The model under review builds one solid part; all positions refer to its coordinate system, in mm. Face numbers are marked on the shaded views. A direction names the side the tool comes from. Round coordinates to 2 decimals unless told otherwise and drop trailing zeros. Write each loop counter-clockwise with the first axis right and the second up, starting at its lowest first coordinate (ties: lowest second). Pieces come first, ordered by that corner, then holes. Notation, with made-up numbers: (-14.75, -16.5) - (43.25, -16.5) arc R22 cw to (43.25, 22.5) - close; hole circle Ø3 at (84, 11.5). An arc over 180 degrees is marked (long way). Return JSON: item names as keys, results as strings.
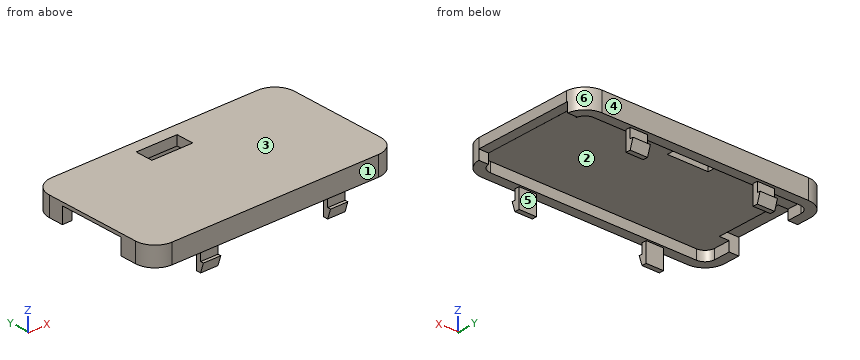
from build123d import *

# Parameters (mm, degrees)
EXTRUDE_1_DEPTH     = 1.5
EXTRUDE_2_DEPTH     = 1.5
CUT_EXTRUDE_2_DEPTH = 1.5
SKETCH_8_W          = 6.342405544
SKETCH_8_H          = 2.722912939
CUT_EXTRUDE_3_DEPTH = 1.5
SKETCH_9_W          = 2.696269273
SKETCH_9_H          = 0.7312398
EXTRUDE_4_DEPTH     = 3
EXTRUDE_6_REACH     = 61.436
CUT_EXTRUDE_4_DEPTH = 17.033846789
SKETCH_6_W          = 3.802870335
SKETCH_6_H          = 10.25
CUT_EXTRUDE_5_DEPTH = 3.024817901


with BuildPart() as part:
    # 草图1 → 凸台-拉伸1 (new body)
    with BuildSketch(Plane.XY.offset(46.24708128)):
        with BuildLine():
            Line((-18.935673231, -7.132078693), (13.064326769, -7.132078693))
            ThreePointArc((13.064326769, -7.132078693), (15.140982735, -6.297142202), (16.061721471, -4.257078693))
            Line((16.061721471, -4.257078693), (16.061721471, 10.992921307))
            ThreePointArc((16.061721471, 10.992921307), (15.140982735, 13.032984817), (13.064326769, 13.867921307))
            Line((13.064326769, 13.867921307), (-18.935673231, 13.867921307))
            ThreePointArc((-18.935673231, 13.867921307), (-21.056993574, 12.989241651), (-21.935673231, 10.867921307))
            Line((-21.935673231, 10.867921307), (-21.935673231, -4.132078693))
            ThreePointArc((-21.935673231, -4.132078693), (-21.056993574, -6.253399036), (-18.935673231, -7.132078693))
        make_face()
        with BuildLine():
            Line((13.064326769, -5.632078693), (-18.935673231, -5.632078693))
            ThreePointArc((-18.935673231, -5.632078693), (-19.996333403, -5.192738865), (-20.435673231, -4.132078693))
            Line((-20.435673231, -4.132078693), (-20.435673231, 10.867921307))
            ThreePointArc((-20.435673231, 10.867921307), (-19.996333403, 11.928581479), (-18.935673231, 12.367921307))
            Line((-18.935673231, 12.367921307), (13.064326769, 12.367921307))
            ThreePointArc((13.064326769, 12.367921307), (14.124986941, 11.928581479), (14.564326769, 10.867921307))
            Line((14.564326769, 10.867921307), (14.564326769, -4.132078693))
            ThreePointArc((14.564326769, -4.132078693), (14.124986941, -5.192738865), (13.064326769, -5.632078693))
        make_face(mode=Mode.SUBTRACT)
    extrude(amount=EXTRUDE_1_DEPTH)

    # 草图4 → 凸台-拉伸2 (add)
    with BuildSketch(Plane.XY.offset(47.74708128)):
        with BuildLine():
            Line((-21.935673231, 10.867921307), (-21.935673231, -4.132078693))
            ThreePointArc((-21.935673231, -4.132078693), (-21.056993574, -6.253399036), (-18.935673231, -7.132078693))
            Line((-18.935673231, -7.132078693), (13.064326769, -7.132078693))
            ThreePointArc((13.064326769, -7.132078693), (15.140982735, -6.297142202), (16.061721471, -4.257078693))
            Line((16.061721471, -4.257078693), (16.061721471, 10.992921307))
            ThreePointArc((16.061721471, 10.992921307), (15.140982735, 13.032984817), (13.064326769, 13.867921307))
            Line((13.064326769, 13.867921307), (-18.935673231, 13.867921307))
            ThreePointArc((-18.935673231, 13.867921307), (-21.056993574, 12.989241651), (-21.935673231, 10.867921307))
        make_face()
    extrude(amount=EXTRUDE_2_DEPTH)

    # 草图7 → 切除-拉伸2 (cut)
    with BuildSketch(Plane(origin=(16.061721471, 0, 0), x_dir=(0, 0, -1), z_dir=(1, 0, 0))):
        Polygon((-46.24708128, 11.189366068), (-47.753743169, 11.189366068), (-47.74708128, -4.257078693), (-46.24708128, -4.257078693), align=None)
    extrude(amount=-CUT_EXTRUDE_2_DEPTH, mode=Mode.SUBTRACT)

    # 草图8 → 切除-拉伸3 (cut)
    with BuildSketch(Plane.XY.offset(49.24708128)):
        with Locations((-4.288714371, 10.645412295)):
            Rectangle(SKETCH_8_W, SKETCH_8_H)
    extrude(amount=-CUT_EXTRUDE_3_DEPTH, mode=Mode.SUBTRACT)

    # 草图9 → 凸台-拉伸4 (add)
    with BuildSketch(Plane(origin=(0, 0, 46.24708128), x_dir=(-1, 0, 0), z_dir=(0, 0, -1))):
        with Locations((-6.965713307, 13.038581452)):
            Rectangle(SKETCH_9_W, SKETCH_9_H)
        with Locations((12.764402756, 13.038581452)):
            Rectangle(SKETCH_9_W, SKETCH_9_H)
        with Locations((12.764402756, -6.302738837)):
            Rectangle(SKETCH_9_W, SKETCH_9_H)
        with Locations((-6.965713307, -6.302738837)):
            Rectangle(SKETCH_9_W, SKETCH_9_H)
    extrude(amount=EXTRUDE_4_DEPTH)

    # 凸台-拉伸6: up to this face of the body (flat: up to its plane)
    extrude_6_end = Plane(part.part.faces().sort_by_distance((-14.112537392, 13.038581452, 44.74708128))[0])
    # 草图10 → 凸台-拉伸6 (add, up to the picked face)
    with BuildSketch(Plane(origin=(8.313847943, 0, 0), x_dir=(0, 0, -1), z_dir=(1, 0, 0)), mode=Mode.PRIVATE) as extrude_6_sk1:
        Polygon((-44.74708128, 13.404201352), (-44.74708128, 13.89248872), (-43.24708128, 13.404201352), align=None)
    extrude_6_tool1 = split(extrude(extrude_6_sk1.sketch, amount=-EXTRUDE_6_REACH, mode=Mode.PRIVATE), bisect_by=extrude_6_end, keep=Keep.BOTH, mode=Mode.PRIVATE)
    extrude_6 = extrude_6_tool1.solids().sort_by(Axis((8.313848, 13.566964, 44.247081), (-1, 0, 0)))[0]
    add(extrude_6)

    # 草图11 → 切除-拉伸4 (cut)
    with BuildSketch(Plane(origin=(-11.416268119, 0, 0), x_dir=(0, 0, -1), z_dir=(1, 0, 0))):
        Polygon((-44.74708128, 13.404201352), (-43.24708128, 13.404201352), (-44.74708128, 13.89248872), align=None)
    cut_extrude_4 = extrude(amount=CUT_EXTRUDE_4_DEPTH, mode=Mode.SUBTRACT)

    # 镜向1: 凸台-拉伸6 across plane
    add(extrude_6.mirror(Plane(origin=(0, 3.367921307, 0), x_dir=(0, 0, 1), z_dir=(0, -1, 0))))

    # 镜向2: 切除-拉伸4 across plane
    add(cut_extrude_4.mirror(Plane(origin=(0, 3.367921307, 0), x_dir=(0, 0, 1), z_dir=(0, -1, 0))), mode=Mode.SUBTRACT)

    # 草图6 → 切除-拉伸5 (cut)
    with BuildSketch(Plane.ZY.offset(21.935673231)):
        with Locations((46.829796448, 3.511921307)):
            Rectangle(SKETCH_6_W, SKETCH_6_H)
    extrude(amount=-CUT_EXTRUDE_5_DEPTH, mode=Mode.SUBTRACT)


solid = part.part
(1) Wall thickness on line 1 (X direction, y = 10.75, z = 48.8); line 2 (Y direction, x = -7.5, z = 47.4); line 3 (Z direction, x = 11.5, y = 4): over which ranges is each line inside the solid? List them lowest first.
Filled in:
{"line 1": "x = -21.94 to -7.46, -1.12 to 16.06", "line 2": "y = -7.13 to -5.63, 12.37 to 13.87", "line 3": "z = 47.75 to 49.25"}
(2) Add section A-A (z = 45.5). Write out the cut boundary in (x, y), plus the area to 3 significant figures.
Filled in:
{"outline": "(-14.11, -6.67) - (-11.42, -6.67) - (-11.42, -5.94) - (-14.11, -5.94) - close; (-14.11, 12.67) - (-11.42, 12.67) - (-11.42, 13.4) - (-14.11, 13.4) - close; (5.62, -6.67) - (8.31, -6.67) - (8.31, -5.94) - (5.62, -5.94) - close; (5.62, 12.67) - (8.31, 12.67) - (8.31, 13.4) - (5.62, 13.4) - close", "area": "7.89 mm2"}
(3) Add section B-B (x = -4.5). Write out the cut boundary in (y, z), plus the area to 3 significant figures.
Filled in:
{"outline": "(-7.13, 46.25) - (-5.63, 46.25) - (-5.63, 47.75) - (9.28, 47.75) - (9.28, 49.25) - (-7.13, 49.25) - close; (12.01, 47.75) - (12.37, 47.75) - (12.37, 46.25) - (13.87, 46.25) - (13.87, 49.25) - (12.01, 49.25) - close", "area": "31.9 mm2"}
(4) For the marked faces 5 and 6, list the 3-axis set-ups (+Z, -Z, +X, -X, +Y, -Y) from which the entire face can be reached by the end or side of a thin tool; tool diameter is ignored.
Filled in:
{"face 5": "-Z, +X, -X", "face 6": "+Z, -Z, +X, +Y"}
(5) Clearance check with flat-ended pins moving along their axes: pin 1 Ø1.6 at (x, y) = (15.5, 0.5) entering from -Z; pin 2 Ø2 at (x, z) = (-13, 45) entering from +Y; pin 3 Ø0.7 at (x, z) = (-21, 48) entering from -Y; pin 4 Ø1.6 at (x, z) = (-2.5, 48.5) entering from -Y. State where each tip first meets the part, or that it passes through.
Filled in:
{"pin 1": "stops at z = 47.75", "pin 2": "stops at y = 13.89", "pin 3": "stops at y = -6.59", "pin 4": "stops at y = -7.13"}
(6) Mouldability with a two-part tool opening along Y and no side actions: class the marked faces 1, 2, 3 and 4 as released by +Y, released by -Y, zero draft, split by the parting line, or undercut.
Filled in:
{"face 1": "released by -Y", "face 2": "undercut", "face 3": "zero draft", "face 4": "released by +Y"}
(7) Add section D-D (x = -16.5). Write out the cut boundary in (y, z).
Filled in:
{"outline": "(-7.13, 46.25) - (-5.63, 46.25) - (-5.63, 47.75) - (12.37, 47.75) - (12.37, 46.25) - (13.87, 46.25) - (13.87, 49.25) - (-7.13, 49.25) - close"}
